Can you work these out from the model? Positions are in its coordinate system, mm. A direction names the side the tool comes from. Give positions to 0.01 mm unless a question says otherwise; leave off trailing zeros. Write each loop counter-clockwise with the first axis right and the second up, starting at its lowest first coordinate (ties: lowest second). Pieces come first, ordered by that corner, then holes.
from build123d import *

# Parameters (mm, degrees)
SKETCH1_W           = 22.5
SKETCH1_H           = 30
SKETCH1_W_2         = 7.5
SKETCH1_H_2         = 7.5
BOSS_EXTRUDE1_DEPTH = 5
CUT_EXTRUDE1_DEPTH  = 51.698249477


with BuildPart() as part:
    # Sketch1 → Boss-Extrude1 (new body)
    with BuildSketch(Plane(origin=(0, 0, 0), x_dir=(1, 0, 0), z_dir=(0, 1, 0))):
        Polygon((-11.25, 7.5), (-11.25, 15), (-26.25, 15), (-26.25, -15), (-18.75, -15), (-18.75, 7.5), align=None)
        Rectangle(SKETCH1_W, SKETCH1_H)
        with Locations((0, 18.75)):
            Rectangle(SKETCH1_W_2, SKETCH1_H_2)
        Polygon((26.25, 15), (11.25, 15), (11.25, 7.5), (33.75, 7.5), (33.75, 22.5), (26.25, 22.5), align=None)
        Polygon((26.25, -7.5), (11.25, -7.5), (11.25, -15), (18.75, -15), (18.75, -30), (33.75, -30), (33.75, -22.5), (26.25, -22.5), align=None)
        Polygon((-3.75, -22.5), (-3.75, -15), (-11.25, -15), (-11.25, -30), (3.75, -30), (3.75, -37.5), (11.25, -37.5), (11.25, -22.5), align=None)
    extrude(amount=BOSS_EXTRUDE1_DEPTH)

    # Sketch2 → Cut-Extrude1 (cut, through all)
    with BuildSketch(Plane(origin=(0, 5, 0), x_dir=(1, 0, 0), z_dir=(0, 1, 0))):
        Polygon((-5.773502692, 5), (5.773502692, 5), (0, -5), align=None)
    extrude(amount=-CUT_EXTRUDE1_DEPTH, mode=Mode.SUBTRACT)


solid = part.part
(1) Imagine slicing it at D-D, the plane z = 0. Write out the boundary of the cut face in (x, y).
Returned:
outline: (-26.25, 0) - (-18.75, 0) - (-18.75, 5) - (-26.25, 5) - close; (-11.25, 0) - (-2.89, 0) - (-2.89, 5) - (-11.25, 5) - close; (2.89, 0) - (11.25, 0) - (11.25, 5) - (2.89, 5) - close
(2) Imagine slicing it at A-A, the plane x = 16. Write out the boundary of the cut face in (y, z).
Returned:
outline: (0, -15) - (5, -15) - (5, -7.5) - (0, -7.5) - close; (0, 7.5) - (5, 7.5) - (5, 15) - (0, 15) - close
(3) If we mould it in two halves opening along Z, with no side actions, what happens to faces 1 (the face through (7, 2, 37.5)), 2 (the face through (4, 2, 22.5)), 3 (the face through (-11.25, 2, 11)), 4 (the face through (-15, 2, -15))? For each: +Z half, -Z half, draft (parallel to the pull), parting line (faces both ways), or undercut.
Returned:
face 1: +Z half
face 2: undercut
face 3: draft
face 4: -Z half
(4) If I drill on L1, parallel to Z at x = 21.5, y = 2.5; L2, parallel to Z at x = 26.5, y = 3.7; L3, parallel to X at y = 0.4, z = 25, over which ranges is the centre line in solid material (lowest first)?
Returned:
L1: z = -15 to -7.5, 7.5 to 30
L2: z = -22.5 to -7.5, 22.5 to 30
L3: x = -11.25 to 11.25, 18.75 to 33.75
(5) Will these pins go through, and if not, where does the flat tip stop? P1, Ø1.5, axis at x = -24, y = 3.5, coming from the +Z side; P2, Ø1.5, axis at y = 1.5, z = -19.5, coming from the -X side; P3, Ø2.5, axis at y = 3.5, z = 7.5, coming from the +X side.
Returned:
P1: stops at z = 15
P2: stops at x = -3.75
P3: stops at x = 26.25
(6) For faces 5 (the face through (7, 2, 15)), 6 (the face through (-18.75, 2, 4)), 7 (the face through (22, 2, -7.5)), which set-ups out of +Z, -Z, +X, -X, +Y, -Y let a thin tool reach every point of the face, with its end or its side?
Returned:
face 5: +Y, -Y
face 6: +Z, +Y, -Y
face 7: +X, +Y, -Y
(7) Imagine slicing it at B-B, the plane z = -6. Write out the boundary of the cut face in (x, y), plus the area to 3 significant figures.
Returned:
outline: (-26.25, 0) - (-18.75, 0) - (-18.75, 5) - (-26.25, 5) - close; (-11.25, 0) - (11.25, 0) - (11.25, 5) - (-11.25, 5) - close
area: 150 mm2
